Source: CAD feature listing. Evaluate the final solid. Frame: model axes, mm. Face numbers are marked on the shaded views. Round coordinates to 2 decimals unless told otherwise and drop trailing zeros. Order: outer loops, then holes, each group sorted by start corner. A loop starts at its lowest first (then second) coordinate and runs counter-clockwise, first axis right, second up.
```python
from build123d import *


with BuildPart() as part:
    # Sketch2 → Revolve1 (revolve)
    with BuildSketch(Plane(origin=(0, 0, 0), x_dir=(0, 0, -1), z_dir=(1, 0, 0))):
        with BuildLine():
            Line((-12.7, -5.55625), (-12.7, 5.55625))
            Line((-12.7, 5.55625), (-17.4625, 5.55625))
            ThreePointArc((-17.4625, 5.55625), (-20.830096045, 4.161346045), (-22.225, 0.79375))
            Line((-22.225, 0.79375), (-17.4625, 0.79375))
            Line((-17.4625, 0.79375), (-17.4625, -0.79375))
            Line((-17.4625, -0.79375), (-22.225, -0.79375))
            ThreePointArc((-22.225, -0.79375), (-20.830096045, -4.161346045), (-17.4625, -5.55625))
            Line((-17.4625, -5.55625), (-12.7, -5.55625))
        make_face()
    revolve(axis=Axis((0, -5.55625, 0), (0, 1, 0)))


solid = part.part
```
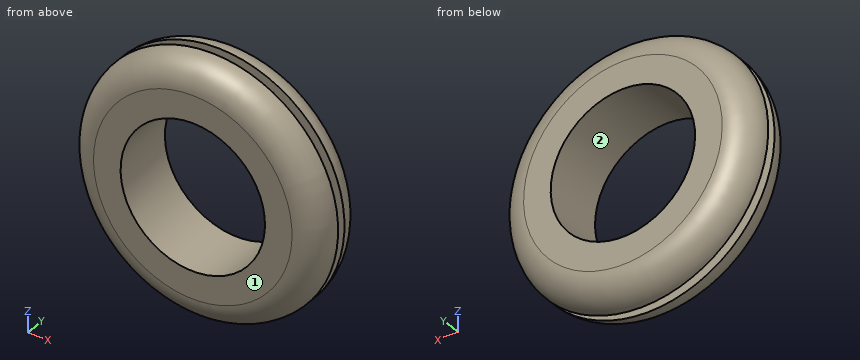
1. First-contact query: pin 1 (1 mm diameter, centred on y = -3, z = -15, fed in from +X); pin 2 (5 mm diameter, centred on y = -4, z = -2, fed in from +X); pin 3 (5 mm diameter, centred on y = -1.5, z = 5.5, fed in from +X); pin 4 (20.5 mm diameter, centred on x = 0, z = 0, fed in from +Y). Flat tips, straight axial feed; report the tip coordinate or a pass-through.
2. Section B-B on z = 0. Return loops of the section in (x, y) (1 decimal).
3. Line query: line 1 along X through (y, z) = (0, 0); line 2 along Y through (x, z) = (-16.5, -11.5); line 3 along Y through (x, z) = (12, -17.5). Output: solid intervals per line, ascending.
4. Section D-D on y = 1.75. Return loops of the section in (x, z), plus the area to 3 significant figures.
5. Pull-direction query (Z, two-part tool) for the marked faces 1 and 2; classes: released by +Z, released by -Z, zero draft, split by the parting line, or undercut.
6. Section C-C on y = -4. Return loops of the section in (x, z), plus the area to 3 significant figures.
7. Section A-A on x = 0. Return loops of the section in (y, z) (1 decimal), plus the area to 3 significant figures.
Result:
1. pin 1: stops at x = 16.23
1. pin 2: stops at x = 22.12
1. pin 3: stops at x = 22.01
1. pin 4: passes through
2. outline: (-22.2, -0.8) arc R4.8 ccw to (-17.5, -5.6) - (-12.7, -5.6) - (-12.7, 5.6) - (-17.5, 5.6) arc R4.8 ccw to (-22.2, 0.8) - (-17.5, 0.8) - (-17.5, -0.8) - close; (12.7, -5.6) - (17.5, -5.6) arc R4.8 ccw to (22.2, -0.8) - (17.5, -0.8) - (17.5, 0.8) - (22.2, 0.8) arc R4.8 ccw to (17.5, 5.6) - (12.7, 5.6) - close
3. line 1: x = -17.46 to -12.7, 12.7 to 17.46
3. line 2: y = -4.75 to -0.79, 0.79 to 4.75
3. line 3: y = -3.72 to -0.79, 0.79 to 3.72
4. outline: circle Ø44.26 at (0, 0); hole circle Ø25.4 at (0, 0)
4. area: 1,030 mm2
5. face 1: zero draft
5. face 2: undercut
6. outline: circle Ø41.97 at (0, 0); hole circle Ø25.4 at (0, 0)
6. area: 877 mm2
7. outline: (-5.6, -17.5) arc R4.8 ccw to (-0.8, -22.2) - (-0.8, -17.5) - (0.8, -17.5) - (0.8, -22.2) arc R4.8 ccw to (5.6, -17.5) - (5.6, -12.7) - (-5.6, -12.7) - close; (-5.6, 12.7) - (5.6, 12.7) - (5.6, 17.5) arc R4.8 ccw to (0.8, 22.2) - (0.8, 17.5) - (-0.8, 17.5) - (-0.8, 22.2) arc R4.8 ccw to (-5.6, 17.5) - close
7. area: 177 mm2
